from build123d import *

# Parameters (mm, degrees)
SKETCH001_R       = 4
PAD_DEPTH         = 5
SKETCH002_R       = 1.5
POCKET_DEPTH      = 5.001
POCKET_DEPTH_BACK = -5.001


with BuildPart() as part:
    # Sketch (on DatumPlane) → Revolution (revolve)
    with BuildSketch(Plane.XZ):
        Polygon((0, 0), (2, 0), (2, 12), (4, 12), (4, 18), (0, 18), align=None)
    revolve(axis=Axis((0, 0, 0), (0, 0, 1)))

    # Sketch001 (on DatumPlane) → Pad (new body, symmetric)
    with BuildSketch(Plane.XZ):
        with Locations((0, 18)):
            Circle(SKETCH001_R)
    extrude(amount=PAD_DEPTH, both=True)

    # Sketch002 (on DatumPlane) → Pocket (cut, two sides)
    with BuildSketch(Plane.XZ) as pocket_sk:
        with Locations((0, 18)):
            Circle(SKETCH002_R)
    extrude(amount=-POCKET_DEPTH, mode=Mode.SUBTRACT)
    extrude(pocket_sk.sketch, amount=-POCKET_DEPTH_BACK, mode=Mode.SUBTRACT)


solid = part.part
Could you check a few things on this model? Use its own coordinates, in mm. A direction names the side the tool comes from. Round coordinates to 2 decimals unless told otherwise and drop trailing zeros. Order: outer loops, then holes, each group sorted by start corner. A loop starts at its lowest first (then second) coordinate and runs counter-clockwise, first axis right, second up.
(1) Imagine slicing it at D-D (z = 7.5). Write out the boundary of the cut face in (x, y), plus the area to 3 significant figures.
Response values:
outline: circle Ø4 at (0, 0)
area: 12.6 mm2
(2) Which directions (+Z, -Z, +X, -X, +Y, -Y) give clear straight access to the entire face, cutting with the end or side of a thin tool? Please do faces 4 (the flat face through (0, 0, 0)), 5 (the cylindrical face through (-4, 0, 14)).
Response values:
face 4: -Z, +X, -X, +Y, -Y
face 5: -Z
(3) I'm going to push flat-ended pins straight in: pin 1 (6 mm diameter, centred on y = -1.5, z = 7, fed in from -X); pin 2 (2.5 mm diameter, centred on x = 0, z = 18, fed in from -Y); pin 3 (1.5 mm diameter, centred on x = 3, z = 12, fed in from +Y). Where does each tip first touch, or does it pass through?
Response values:
pin 1: stops at x = -2
pin 2: passes through
pin 3: stops at y = 3.31
(4) Imagine slicing it at C-C (x = 3). Write out the boundary of the cut face in (y, z), plus the area to 3 significant figures.
Response values:
outline: (-5, 15.35) - (-2.65, 15.35) - (-2.65, 12) - (2.65, 12) - (2.65, 15.35) - (5, 15.35) - (5, 20.65) - (-5, 20.65) - close
area: 70.7 mm2
(5) Imagine slicing it at B-B (y = -3.25). Write out the boundary of the cut face in (x, z).
Response values:
outline: (-2.33, 12) - (2.33, 12) - (2.33, 14.75) arc R4 ccw (long way) to (-2.33, 14.75) - close; hole circle Ø3 at (0, 18)
(6) If we mould it in two halves opening along Z, with no side actions, what happens to faces 1 (the flat face through (0, -5, 16)), 2 (the flat face through (2, -1, 12)), 3 (the cylindrical face through (-0.521, -0.07, 21.966))? For each: released by +Z, released by -Z, zero draft, split by the parting line, or undercut.
Response values:
face 1: zero draft
face 2: released by -Z
face 3: split by the parting line
(7) Imagine slicing it at A-A (x = 0). Write out the boundary of the cut face in (y, z), plus the area to 3 significant figures.
Response values:
outline: (-5, 14) - (-4, 14) - (-4, 12) - (-2, 12) - (-2, 0) - (2, 0) - (2, 12) - (4, 12) - (4, 14) - (5, 14) - (5, 16.5) - (-5, 16.5) - close; (-5, 19.5) - (5, 19.5) - (5, 22) - (-5, 22) - close
area: 114 mm2
(8) Please list where these lines run through material, in increasing order: line 1 along Z through (x, y) = (0, 2.55); line 2 along X through (y, z) = (-2.55, 18); line 3 along Z through (x, y) = (0, 4.05).
Response values:
line 1: z = 12 to 16.5, 19.5 to 22
line 2: x = -4 to -1.5, 1.5 to 4
line 3: z = 14 to 16.5, 19.5 to 22
